Could you check a few things on this model? Use its own coordinates, in mm. A direction names the side the tool comes from. Round coordinates to 2 decimals unless told otherwise and drop trailing zeros. Write each loop counter-clockwise with the first axis right and the second up, starting at its lowest first coordinate (ties: lowest second). Pieces come first, ordered by that corner, then holes.
```python
from build123d import *

# Parameters (mm, degrees)
SKETCH1_W           = 27.3
SKETCH1_H           = 36.4
SKETCH1_W_2         = 10.2
SKETCH1_H_2         = 25
BOSS_EXTRUDE1_DEPTH = 5
SKETCH2_R           = 1.75
CUT_EXTRUDE1_DEPTH  = 5


with BuildPart() as part:
    # Sketch1 → Boss-Extrude1 (new body)
    with BuildSketch(Plane.XY):
        Rectangle(SKETCH1_W, SKETCH1_H)
        Rectangle(SKETCH1_W_2, SKETCH1_H_2, mode=Mode.SUBTRACT)
    extrude(amount=BOSS_EXTRUDE1_DEPTH)

    # Sketch2 → Cut-Extrude1 (cut)
    with BuildSketch(Plane.XY.offset(5)):
        with Locations((-9.5, 11)):
            Circle(SKETCH2_R)
        with Locations(Location((9.5, 11, 0), (0, 0, 180))):
            Circle(SKETCH2_R)
        with Locations(Location((-9.5, -11, 0), (0, 0, 180))):
            Circle(SKETCH2_R)
        with Locations((9.5, -11)):
            Circle(SKETCH2_R)
    extrude(amount=-CUT_EXTRUDE1_DEPTH, mode=Mode.SUBTRACT)


solid = part.part
```
Q1. Imagine slicing it at B-B, the plane y = -11. Write out the boundary of the cut face in (x, z), then the cut area to 3 significant figures.
Q2. We'd pull the mould along X, two halves only. Please class faces 1 (the cylindrical face through (-8.6, 12.5, 2.5)), 2 (the flat face through (-13.65, 0, 2)), 3 (the flat face through (-6, 0, 0)), 4 (the flat face through (0, 12.5, 2)): pulls with the +X half, pulls with the -X half, needs draft (parallel to the pull), parting line crosses it, or undercut.
Q3. Imagine slicing it at A-A, the plane x = 3.5. Write out the boundary of the cut face in (y, z).
Q4. Imagine slicing it at D-D, the plane y = 2.5. Write out the boundary of the cut face in (x, z).
Q5. On a 3-axis mill with a long thin cutter (end or side, diameter ignored), from which of +Z, -Z, +X, -X, +Y, -Y can I reach the whole of each face in a straight line? I mean faces 5 (the flat face through (0, 18.2, 2)), 6 (the flat face through (0, -12.5, 2)). Say none if no direction works.
Q6. Imagine slicing it at C-C, the plane x = -9.5. Write out the boundary of the cut face in (y, z), then the cut area to 3 significant figures.
Q7. If I drill on L1, parallel to Y at x = -9.5, z = 2.4; L2, parallel to X at y = 6.5, z = 3.4; L3, parallel to Y at x = 0, z = 2.05, over which ranges is the centre line in solid material (lowest first)?
Results found:
1. outline: (-13.65, 0) - (-11.25, 0) - (-11.25, 5) - (-13.65, 5) - close; (-7.75, 0) - (-5.1, 0) - (-5.1, 5) - (-7.75, 5) - close; (5.1, 0) - (7.75, 0) - (7.75, 5) - (5.1, 5) - close; (11.25, 0) - (13.65, 0) - (13.65, 5) - (11.25, 5) - close
1. area: 50.5 mm2
2. face 1: undercut
2. face 2: pulls with the -X half
2. face 3: needs draft
2. face 4: undercut
3. outline: (-18.2, 0) - (-12.5, 0) - (-12.5, 5) - (-18.2, 5) - close; (12.5, 0) - (18.2, 0) - (18.2, 5) - (12.5, 5) - close
4. outline: (-13.65, 0) - (-5.1, 0) - (-5.1, 5) - (-13.65, 5) - close; (5.1, 0) - (13.65, 0) - (13.65, 5) - (5.1, 5) - close
5. face 5: +Z, -Z, +X, -X, +Y
5. face 6: +Z, -Z
6. outline: (-18.2, 0) - (-12.75, 0) - (-12.75, 5) - (-18.2, 5) - close; (-9.25, 0) - (9.25, 0) - (9.25, 5) - (-9.25, 5) - close; (12.75, 0) - (18.2, 0) - (18.2, 5) - (12.75, 5) - close
6. area: 147 mm2
7. L1: y = -18.2 to -12.75, -9.25 to 9.25, 12.75 to 18.2
7. L2: x = -13.65 to -5.1, 5.1 to 13.65
7. L3: y = -18.2 to -12.5, 12.5 to 18.2
